Check sheet for the modelled part. Datum: model origin and axes. Units: mm. A direction names the side the tool comes from. Coordinates: 2 decimals unless noted, no trailing zeros. Loops run counter-clockwise (first coordinate to the right, second up) from the corner with the lowest first, then second, coordinate; pieces in that order, holes last. Notation, with made-up numbers: M 33,-11 L 70,-11 A21 ccw 70,25 Z; hole C 49,18 d1. An arc over 180 degrees is marked long. Use CSV: the item, a comma, the result in double quotes. Start each with the question number.
(1) Draft check along Z on faces 4 (the flat face through (-3.859, 5.559, 0.507)), 5 (the flat face through (2.406, 25, 20)), 6 (the cylindrical face through (-3.3, 33.16, 29.77)). Enter one of: pulls with the +Z half, pulls with the -Z half, needs draft (parallel to the pull), parting line crosses it, or undercut.
(2) Section check A-A on z = 37.5. Record the cut outline in (x, y).
(3) Go/stop test with flat-tipped pins: pin 1 Ø4 at (x, z) = (-3.59, 32) entering from +Y; pin 2 Ø6 at (x, z) = (-43, 29) entering from -Y; pin 3 Ø6 at (x, z) = (-41, 28.5) entering from -Y; pin 4 Ø7 at (x, z) = (-43.59, 32) entering from +Y. Record where each tip stops, or that it passes through.
(4) Section check B-B on z = 13.5. Record the cut outline in (x, y), and give its area (3 significant figures).
(5) Set-up check for faces 1 (the cylindrical face through (-45.74, 33.16, 31.32)), 2 (the flat face through (-23, -0.873, 20)), 3 (the cylindrical face through (-11.82, 35.29, 36.9)): record each of +Z, -Z, +X, -X, +Y, -Y from which the full face is reachable in a straight line by a thin tool's end or side.
(6) Scan lines: line 1 (X direction, y = 36, z = 8); line 2 (X direction, y = 32.25, z = 8); line 3 (X direction, y = 30.5, z = 32). Record each from-to range of solid material in increasing order.
from build123d import *

# Parameters (mm, degrees)
BOSS_EXTRUDE1_DEPTH             = 40
SKETCH2_R                       = 14
CUT_EXTRUDE1_DEPTH              = 40
M5X0_5_TAPPED_HOLE4_D           = 4.5
M5X0_5_TAPPED_HOLE4_DEPTH       = 11.5
M5X0_5_TAPPED_HOLE4_CSINK_D     = 5.05
M5X0_5_TAPPED_HOLE4_CSINK_ANGLE = 90
M5X0_5_TAPPED_HOLE4_TIP         = 1.351936393
CIRPATTERN1_COUNT               = 8
CHAMFER1_SIZE                   = 1
CHAMFER2_SIZE                   = 1


with BuildPart() as part:
    # Sketch1 → Boss-Extrude1 (new body)
    with BuildSketch(Plane.XY):
        Polygon((-49.594358144, 39.126859892), (2.405641856, 39.126859892), (2.405641856, 11.126859892), (-9.594358144, -0.873140108), (-37.594358144, -0.873140108), (-49.594358144, 11.126859892), align=None)
    extrude(amount=BOSS_EXTRUDE1_DEPTH)

    # Sketch2 → Cut-Extrude1 (cut)
    with BuildSketch(Plane.XY.offset(40)):
        with Locations((-24.558993323, 19.837643708)):
            Circle(SKETCH2_R)
    extrude(amount=-CUT_EXTRUDE1_DEPTH, mode=Mode.SUBTRACT)

    # M5x0.5 Tapped Hole4
    with Locations(Plane(origin=(0, 39.126859892, 0), x_dir=(1, 0, 0), z_dir=(0, 1, 0))):
        with Locations((-43.594358144, -32), (-3.594358144, -32), (-3.594358144, -8), (-43.594358144, -8)):
            CounterSinkHole(M5X0_5_TAPPED_HOLE4_D / 2, M5X0_5_TAPPED_HOLE4_CSINK_D / 2, depth=M5X0_5_TAPPED_HOLE4_DEPTH, counter_sink_angle=M5X0_5_TAPPED_HOLE4_CSINK_ANGLE)
            with Locations((0, 0, -(M5X0_5_TAPPED_HOLE4_DEPTH + M5X0_5_TAPPED_HOLE4_TIP / 2))):  # 118° drill point
                Cone(0, M5X0_5_TAPPED_HOLE4_D / 2, M5X0_5_TAPPED_HOLE4_TIP, mode=Mode.SUBTRACT)

    # Sketch15 → M5x0.5 Tapped Hole5 (revolve, cut)
    with BuildSketch(Plane(origin=(-42.594358144, 19.126859892, 40), x_dir=(0, -1, 0), z_dir=(1, 0, 0))):
        Polygon((0, 0), (0, 7.351936393), (2.25, 6), (2.25, 0.275), (2.525, 0), align=None)
    m5x0_5_tapped_hole5 = revolve(axis=Axis((-42.594358144, 19.126859892, 46.35), (0, 0, -1)), mode=Mode.SUBTRACT)

    # CirPattern1: M5x0.5 Tapped Hole5 ×8 about axis, 2 skipped
    cirpattern1_axis = Axis((-24.558993323, 19.837643708, 0), (0, 0, 1))
    add([m5x0_5_tapped_hole5.rotate(cirpattern1_axis, i * 360 / CIRPATTERN1_COUNT) for i in range(1, CIRPATTERN1_COUNT) if i not in (2, 6)], mode=Mode.SUBTRACT)

    # Chamfer1
    chamfer1_edges = [part.edges().sort_by_distance(p)[0] for p in [
        (-23.594358144, -0.873140108, 40),
        (-3.594358144, 5.126859892, 40),
        (2.405641856, 25.126859892, 40),
        (-23.594358144, 39.126859892, 40),
        (-49.594358144, 25.126859892, 40),
        (-23.594358144, 39.126859892, 0),
        (2.405641856, 25.126859892, 0),
        (-3.594358144, 5.126859892, 0),
        (-23.594358144, -0.873140108, 0),
        (-43.594358144, 5.126859892, 0),
        (-49.594358144, 25.126859892, 0),
        (-43.594358144, 5.126859892, 40),
    ]]
    chamfer(chamfer1_edges, length=CHAMFER1_SIZE)

    # Chamfer2
    chamfer2_edges = [part.edges().sort_by_distance(p)[0] for p in [
        (-38.558993323, 19.837643708, 0),
        (-38.558993323, 19.837643708, 40),
    ]]
    chamfer(chamfer2_edges, length=CHAMFER2_SIZE)


solid = part.part
Outcome:
1,face 4,"pulls with the -Z half"
1,face 5,"needs draft"
1,face 6,"undercut"
2,outline,"M -49.59,11.13 L -37.59,-0.87 L -9.59,-0.87 L 2.41,11.13 L 2.41,39.13 L -49.59,39.13 Z; hole C -42.59,19.13 d4.5; hole C -37.81,32.09 d4.5; hole C -36.81,6.58 d4.5; hole C -24.56,19.84 d28; hole C -12.31,33.09 d4.5; hole C -11.3,7.59 d4.5; hole C -6.52,20.55 d4.5"
3,pin 1,"stops at y = 27.48"
3,pin 2,"stops at y = 1.53"
3,pin 3,"stops at y = -0.47"
3,pin 4,"stops at y = 39.13"
4,outline,"M -49.59,11.13 L -37.59,-0.87 L -9.59,-0.87 L 2.41,11.13 L 2.41,39.13 L -49.59,39.13 Z; hole C -24.56,19.84 d28"
4,area,"1,320 mm²"
5,face 1,"+Y"
5,face 2,"+Z, -Z, +X, -X, -Y"
5,face 3,"+Z"
6,line 1,"x = -49.59 to -45.84, -41.34 to -5.84, -1.34 to 2.41"
6,line 2,"x = -49.59 to -45.84, -41.34 to -31.03, -18.08 to -5.84, -1.34 to 2.41"
6,line 3,"x = -49.59 to -45.84, -41.34 to -33.63, -15.49 to -5.84, -1.34 to 2.41"
